CAD build for the part. Positions are in the model's coordinates, mm. Face numbers are marked on the shaded views. A direction names the side the tool comes from. Give positions to 0.01 mm unless a question says otherwise; leave off trailing zeros. Write each loop counter-clockwise with the first axis right and the second up, starting at its lowest first coordinate (ties: lowest second). Pieces come first, ordered by that corner, then holes. Notation, with made-up numbers: (-7.5, 2) -> (-0.5, 2) arc R20 ccw to (-0.5, 40) -> close; hole circle Ø6 at (28.25, -28). An arc over 180 degrees is marked (long way). Use one line per item in the form item = value. Start each with the question number.
from build123d import *

# Parameters (mm, degrees)
BOSS_EXTRUDE1_DEPTH = 6.4008
SKETCH1_3_W         = 1.0541
SKETCH1_3_H         = 1.0922
SKETCH1_3_W_2       = 3.3909
SKETCH1_3_W_3       = 11.049
SKETCH1_3_W_4       = 17.8308
SKETCH1_3_H_2       = 1.524
BOSS_EXTRUDE2_DEPTH = 19.939
SKETCH1_4_W         = 11.049
SKETCH1_4_H         = 2.6162
CUT_EXTRUDE1_DEPTH  = 3.0734
SKETCH2_R           = 7.874
BOSS_EXTRUDE3_DEPTH = 9.4742
CUT_EXTRUDE2_START  = -10.16
CUT_EXTRUDE2_DEPTH  = 10.16


# Read off the part's stored shape, not the designer's step: Cut-Extrude2
with BuildPart() as part:
    # Sketch1 → Boss-Extrude1 (new body)
    with BuildSketch(Plane(origin=(0, 0, 0), x_dir=(1, 0, 0), z_dir=(0, 1, 0))):
        Polygon((1.678214286, -1.50495), (5.069114286, -1.50495), (5.069114286, 8.40105), (-12.761685714, 8.40105), (-12.761685714, -1.50495), (-9.370785714, -1.50495), (-9.370785714, -4.12115), (1.678214286, -4.12115), align=None)
    extrude(amount=BOSS_EXTRUDE1_DEPTH)

    # Sketch1_3 → Boss-Extrude2 (add)
    with BuildSketch(Plane(origin=(0, 0, 0), x_dir=(1, 0, 0), z_dir=(0, 1, 0))):
        with Locations((-13.288735714, -3.57505)):
            Rectangle(SKETCH1_3_W, SKETCH1_3_H)
        with Locations((-11.066235714, -3.57505)):
            Rectangle(SKETCH1_3_W_2, SKETCH1_3_H)
        with Locations((-3.846285714, -3.57505)):
            Rectangle(SKETCH1_3_W_3, SKETCH1_3_H)
        with Locations((3.373664286, -3.57505)):
            Rectangle(SKETCH1_3_W_2, SKETCH1_3_H)
        with Locations((5.596164286, -3.57505)):
            Rectangle(SKETCH1_3_W, SKETCH1_3_H)
        with Locations((-3.846285714, -2.26695)):
            Rectangle(SKETCH1_3_W_4, SKETCH1_3_H_2)
    extrude(amount=BOSS_EXTRUDE2_DEPTH)

    # Sketch1_4 → Cut-Extrude1 (cut)
    with BuildSketch(Plane(origin=(0, 0, 0), x_dir=(1, 0, 0), z_dir=(0, 1, 0))):
        with Locations((-3.846285714, -2.81305)):
            Rectangle(SKETCH1_4_W, SKETCH1_4_H)
    extrude(amount=CUT_EXTRUDE1_DEPTH, mode=Mode.SUBTRACT)

    # Sketch2 → Boss-Extrude3 (add)
    with BuildSketch(Plane(origin=(0, 0, 1.50495), x_dir=(-1, 0, 0), z_dir=(0, 0, -1))):
        with Locations((3.846285714, 9.6774)):
            Circle(SKETCH2_R)
    extrude(amount=BOSS_EXTRUDE3_DEPTH)

    # Cut-Extrude2 outline → Cut-Extrude2 (cut)
    with BuildSketch(Plane.XY.offset(4.12115).offset(CUT_EXTRUDE2_START)):
        with BuildLine():
            ThreePointArc((-2.831556509, 3.0734), (-3.846285715, 16.5862), (-4.86101492, 3.0734))
            Line((-4.86101492, 3.0734), (-2.831556509, 3.0734))
        make_face()
    extrude(amount=CUT_EXTRUDE2_DEPTH, mode=Mode.SUBTRACT)


solid = part.part
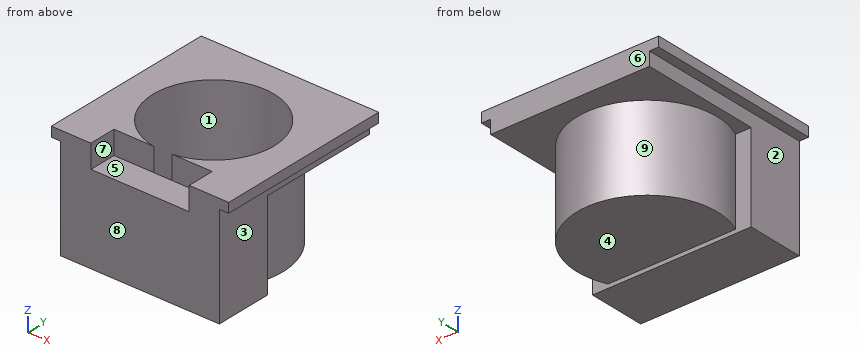
1) Cut at A-A (y = 18). Give the cut face in (x, z), and give its area (3 significant figures).
2) Wall check: line 1 along X through (y, z) = (9.5, -0.75); line 2 along Z through (x, y) = (-0.5, 1); line 3 along Y through (x, z) = (5, -8). Give the ranges that are in metal, low to high. Write a range as from..to.
3) Cut at D-D (y = 2.5). Give the cut face in (x, z).
4) 3-axis set-ups, long thin cutter, end or side, ignore diameter. For the marked faces 1, 2, 3, 4 and 5: which of +Z, -Z, +X, -X, +Y, -Y reach the whole face in a straight line?
5) Pin check, flat tips, straight feed: pin 1 (3 mm diameter, centred on y = 10, z = -6, fed in from -X); pin 2 (0.6 mm diameter, centred on x = -4, z = -3.5, fed in from +Y); pin 3 (1.5 mm diameter, centred on y = 14, z = -1, fed in from +X); pin 4 (3 mm diameter, centred on x = -6, z = 1, fed in from -Y). Stop position of each tip, or through.
6) Cut at C-C (x = -6). Give the cut face in (y, z), and give its area (3 significant figures).
7) Two-plate mould, pull along Y, no slides. Class the marked faces 6, 7, 8 and 9: released by +Y, released by -Y, zero draft, split by the parting line, or undercut.
8) Cut at B-B (z = 2.5). Give the cut face in (x, y), and give its area (3 significant figures).
Final values:
q1.outline = (-13.82, 3.03) -> (-12.76, 3.03) -> (-12.76, 1.5) -> (5.07, 1.5) -> (5.07, 3.03) -> (6.12, 3.03) -> (6.12, 4.12) -> (-13.82, 4.12) -> close
q1.area = 49.0 mm^2
q2.line_1 = -11.72..-10.63, 2.94..4.03
q2.line_2 = -8.4..1.5
q2.line_3 = 0..6.4
q3.outline = (-13.82, 3.03) -> (-12.76, 3.03) -> (-12.76, -8.4) -> (5.07, -8.4) -> (5.07, 3.03) -> (6.12, 3.03) -> (6.12, 4.12) -> (1.68, 4.12) -> (1.68, 1.5) -> (-9.37, 1.5) -> (-9.37, 4.12) -> (-13.82, 4.12) -> close
q4.face_1 = +Z
q4.face_2 = -Z, -X, +Y, -Y
q4.face_3 = -Z, +X, +Y, -Y
q4.face_4 = -Z, +X, -X, +Y
q4.face_5 = +Z, -Y
q5.pin_1 = -11.72
q5.pin_2 = 17.55
q5.pin_3 = 3.17
q5.pin_4 = 0
q6.outline = (0, -8.4) -> (6.4, -8.4) -> (6.4, -7.97) -> (17.25, -7.97) -> (17.25, 1.5) -> (19.94, 1.5) -> (19.94, 4.12) -> (16.24, 4.12) -> (16.24, -6.04) -> (3.35, -6.04) -> (3.35, 4.12) -> (3.07, 4.12) -> (3.07, 1.5) -> (0, 1.5) -> close
q6.area = 79.4 mm^2
q7.face_6 = released by +Y
q7.face_7 = zero draft
q7.face_8 = released by -Y
q7.face_9 = undercut
q8.outline = (-12.76, 0) -> (-9.37, 0) -> (-9.37, 3.07) -> (-4.86, 3.07) arc R6.79 cw (long way) to (-2.83, 3.07) -> (1.68, 3.07) -> (1.68, 0) -> (5.07, 0) -> (5.07, 19.94) -> (-12.76, 19.94) -> close
q8.area = 177 mm^2
